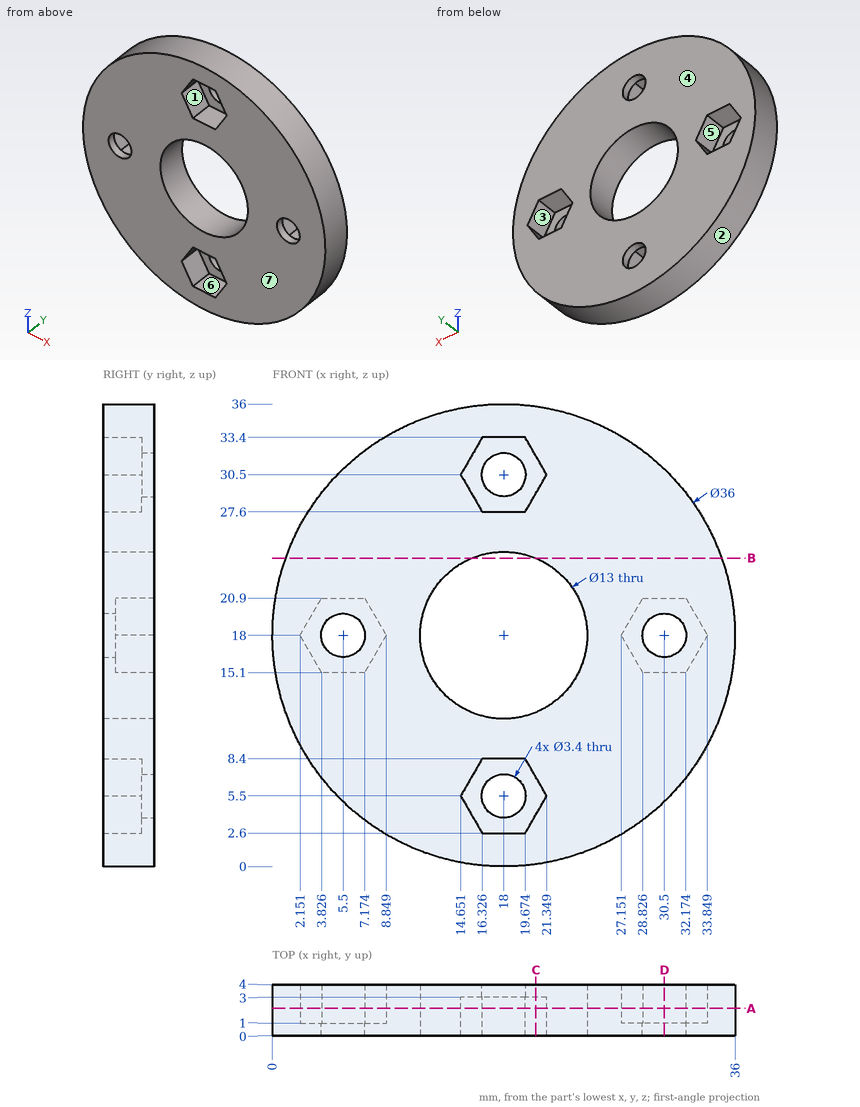
Job drawing, mm, ordinate dimensions from the low corner. One solid piece. A direction names the side the tool comes from. Coordinates: 2 decimals unless noted, no trailing zeros. Order: outer loops, then holes, each group sorted by start corner. A loop starts at its lowest first (then second) coordinate and runs counter-clockwise, first axis right, second up. Notation, with made-up numbers: M 76.25,28.5 L 118.25,28.5 A11 ccw 118.25,42.5 Z; hole C 49.25,61 d8. An arc over 180 degrees is marked long. Answer as CSV lines item,"result".
(1) Band-saw the part on C-C, the plane x = 20.5. List the corners of the cut face in (y, z) (1 decimal).
Geometry says:
outline,"M 0,0.2 L 4,0.2 L 4,12 L 0,12 L 0,7 L 3,7 L 3,4 L 0,4 Z; M 0,24 L 4,24 L 4,35.8 L 0,35.8 L 0,32 L 3,32 L 3,29 L 0,29 Z"
(2) Flat gauge pins, fed straight in: pin 1 (2 mm diameter, centred on x = 18, z = 30.5, fed in from +Y); pin 2 (1 mm diameter, centred on y = 2, z = 27.5, fed in from +X); pin 3 (1 mm diameter, centred on x = 11.5, y = 1.5, fed in from -Z); pin 4 (2 mm diameter, centred on y = 3.5, z = 13, fed in from +X). Where does each tip first touch, or does it go through?
Geometry says:
pin 1,"passes through"
pin 2,"stops at x = 33.59"
pin 3,"stops at z = 1.03"
pin 4,"stops at x = 35.55"
(3) 3-axis set-ups, long thin cutter, end or side, ignore diameter. For the marked faces 5, 6 and 7: which of +Z, -Z, +X, -X, +Y, -Y reach the whole face in a straight line?
Geometry says:
face 5,"+Y"
face 6,"-Y"
face 7,"+Z, -Z, +X, -X, -Y"
(4) Band-saw the part on B-B, the plane z = 24. List the corners of the cut face in (x, y), then the cut area to 3 significant figures.
Geometry says:
outline,"M 1.03,0 L 15.5,0 L 15.5,4 L 1.03,4 Z; M 20.5,0 L 34.97,0 L 34.97,4 L 20.5,4 Z"
area,"116 mm2"
(5) Wall check: line 1 along X through (y, z) = (0.4, 18); line 2 along Z through (x, y) = (20, 0.4) (1 decimal); line 3 along X through (y, z) = (2.6, 23.5) (1 decimal). Give the ranges that are in metal, low to high.
Geometry says:
line 1,"x = 0 to 3.8, 7.2 to 11.5, 24.5 to 28.8, 32.2 to 36"
line 2,"z = 0.1 to 3.2, 7.8 to 11.8, 24.2 to 28.2, 32.8 to 35.9"
line 3,"x = 0.9 to 14.5, 21.5 to 35.1"
(6) Band-saw the part on A-A, the plane y = 2.15. List the corners of the cut face in (x, z) (1 decimal).
Geometry says:
outline,"C 18,18 d36; hole M 2.2,18 L 3.8,15.1 L 7.2,15.1 L 8.8,18 L 7.2,20.9 L 3.8,20.9 Z; hole C 18,18 d13; hole M 14.7,5.5 L 16.3,2.6 L 19.7,2.6 L 21.3,5.5 L 19.7,8.4 L 16.3,8.4 Z; hole M 14.7,30.5 L 16.3,27.6 L 19.7,27.6 L 21.3,30.5 L 19.7,33.4 L 16.3,33.4 Z; hole M 27.2,18 L 28.8,15.1 L 32.2,15.1 L 33.8,18 L 32.2,20.9 L 28.8,20.9 Z"
(7) Pull direction Z, two halves, no side cores. Call the marked faces 1, 2, 3 and 4: +Z half, -Z half, draft (parallel to the pull), parting line (faces both ways), or undercut.
Geometry says:
face 1,"undercut"
face 2,"parting line"
face 3,"undercut"
face 4,"draft"
(8) Band-saw the part on D-D, the plane x = 30.5. List the corners of the cut face in (y, z).
Geometry says:
outline,"M 0,5.05 L 4,5.05 L 4,15.1 L 1,15.1 L 1,16.3 L 0,16.3 Z; M 0,19.7 L 1,19.7 L 1,20.9 L 4,20.9 L 4,30.95 L 0,30.95 Z"
